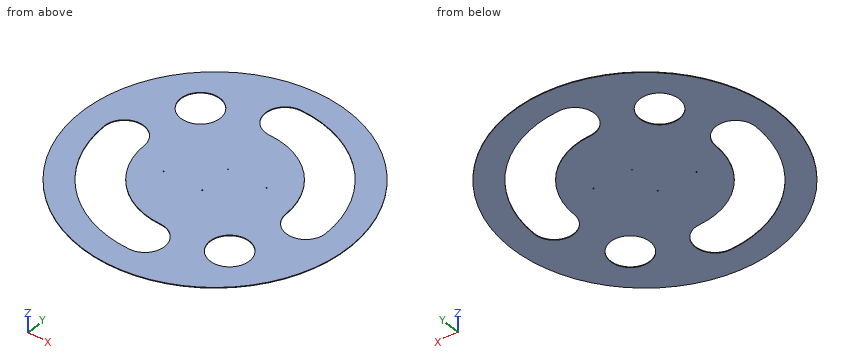
```python
from build123d import *

# Parameters (mm, degrees)
SKETCH_1_R      = 400
SKETCH_1_R_2    = 1.5
SKETCH_1_R_3    = 59
EXTRUDE_1_DEPTH = 2


with BuildPart() as part:
    # 草图1 → 凸台-拉伸1 (new body)
    with BuildSketch(Plane.XY):
        Circle(SKETCH_1_R)
        with Locations((0, -49)):
            Circle(SKETCH_1_R_2, mode=Mode.SUBTRACT)
        with Locations((0, 49)):
            Circle(SKETCH_1_R_2, mode=Mode.SUBTRACT)
        with Locations((-113.5, -49)):
            Circle(SKETCH_1_R_2, mode=Mode.SUBTRACT)
        with Locations((113.5, 49)):
            Circle(SKETCH_1_R_2, mode=Mode.SUBTRACT)
        with Locations((-188.645478562, 188.645478562)):
            Circle(SKETCH_1_R_3, mode=Mode.SUBTRACT)
        with Locations((188.645478562, -188.645478562)):
            Circle(SKETCH_1_R_3, mode=Mode.SUBTRACT)
        with BuildLine():
            ThreePointArc((-325.763672953, 0), (-230.349702209, -230.349702209), (0, -325.763672953))
            ThreePointArc((0, -325.763672953), (58.97867869, -266.784994263), (0, -207.806315572))
            ThreePointArc((0, -207.806315572), (-146.941254915, -146.941254915), (-207.806315572, 0))
            ThreePointArc((-207.806315572, 0), (-266.784994263, 58.97867869), (-325.763672953, 0))
        make_face(mode=Mode.SUBTRACT)
        with BuildLine():
            ThreePointArc((0, 325.763672953), (230.349702209, 230.349702209), (325.763672953, 0))
            ThreePointArc((325.763672953, 0), (266.784994263, -58.97867869), (207.806315572, 0))
            ThreePointArc((207.806315572, 0), (146.941254915, 146.941254915), (0, 207.806315572))
            ThreePointArc((0, 207.806315572), (-58.97867869, 266.784994263), (0, 325.763672953))
        make_face(mode=Mode.SUBTRACT)
    extrude(amount=EXTRUDE_1_DEPTH)


solid = part.part
```
Check sheet for the modelled part. Datum: model origin and axes. Units: mm. Round coordinates to 2 decimals unless told otherwise and drop trailing zeros. Order: outer loops, then holes, each group sorted by start corner. A loop starts at its lowest first (then second) coordinate and runs counter-clockwise, first axis right, second up.
1) Section check A-A (x = 43). Record the boundary of the cut face in (y, z), and give its area (3 significant figures).
2) Section check D-D (x = -84.5). Record the boundary of the cut face in (y, z), and give its area (3 significant figures).
3) Scan lines: line 1 (X direction, y = 186, z = 1.55); line 2 (X direction, y = 5, z = 0.3); line 3 (Y direction, x = -113.5, z = 1.45). Record each from-to range of solid material in increasing order.
4) Section check C-C (z = 1.5). Give the number of separate pieces and of enclosed holes in the cut face, and give its area (3 significant figures).
5) Section check B-B (y = 171). Record the boundary of the cut face in (x, z) (3 decimals).
6) Go/stop test with flat-tipped pins: pin 1 Ø4 at (x, y) = (113.5, 49) entering from -Z; pin 2 Ø1.8 at (x, y) = (0, -49) entering from +Z; pin 3 Ø1 at (y, z) = (-166, 0.5) entering from -X. Record where each tip stops, or that it passes through.
Result:
1. outline: (-397.68, 0) - (-307.15, 0) - (-307.15, 2) - (-397.68, 2) - close; (-226.42, 0) - (203.31, 0) - (203.31, 2) - (-226.42, 2) - close; (322.91, 0) - (397.68, 0) - (397.68, 2) - (322.91, 2) - close
1. area: 1,190 mm2
2. outline: (-390.97, 0) - (-314.61, 0) - (-314.61, 2) - (-390.97, 2) - close; (-189.85, 0) - (390.97, 0) - (390.97, 2) - (-189.85, 2) - close
2. area: 1,310 mm2
3. line 1: x = -354.12 to -247.59, -129.7 to 92.67, 267.44 to 354.12
3. line 2: x = -399.97 to -325.55, -208.02 to 207.75, 325.73 to 399.97
3. line 3: y = -383.56 to -305.35, -174.07 to -50.5, -47.5 to 383.56
4. separate pieces: 1
4. enclosed holes: 8
4. area: 360,000 mm2
5. outline: (-361.606, 0) - (-244.945, 0) - (-244.945, 2) - (-361.606, 2) - close; (-132.346, 0) - (118.078, 0) - (118.078, 2) - (-132.346, 2) - close; (277.274, 0) - (361.606, 0) - (361.606, 2) - (277.274, 2) - close
6. pin 1: stops at z = 0
6. pin 2: passes through
6. pin 3: stops at x = -364.16
